```python
from build123d import *

# Parameters (mm, degrees)
SKETCH1_R           = 3.175
BOSS_EXTRUDE1_DEPTH = 27.686
SKETCH2_R           = 3.175
SKETCH2_R_2         = 2.38125
CUT_EXTRUDE1_DEPTH  = 4.318
SKETCH3_R           = 2.38125
SKETCH3_R_2         = 2.2225
CUT_EXTRUDE2_DEPTH  = 0.4572
SKETCH4_R           = 1.5875
CUT_EXTRUDE3_DEPTH  = 56.553754455


with BuildPart() as part:
    # Sketch1 → Boss-Extrude1 (new, symmetric)
    with BuildSketch(Plane.XY):
        Circle(SKETCH1_R)
    extrude(amount=BOSS_EXTRUDE1_DEPTH, both=True)

    # Sketch2 → Cut-Extrude1 (cut)
    with BuildSketch(Plane.XY.offset(27.686)):
        Circle(SKETCH2_R)
        Circle(SKETCH2_R_2, mode=Mode.SUBTRACT)
    cut_extrude1 = extrude(amount=-CUT_EXTRUDE1_DEPTH, mode=Mode.SUBTRACT)

    # Sketch3 → Cut-Extrude2 (cut)
    with BuildSketch(Plane.XY.offset(26.797)):
        Circle(SKETCH3_R)
        Circle(SKETCH3_R_2, mode=Mode.SUBTRACT)
    cut_extrude2 = extrude(amount=-CUT_EXTRUDE2_DEPTH, mode=Mode.SUBTRACT)

    # Sketch4 → Cut-Extrude3 (cut, through all)
    with BuildSketch(Plane.XY.offset(27.686)):
        Circle(SKETCH4_R)
    extrude(amount=-CUT_EXTRUDE3_DEPTH, mode=Mode.SUBTRACT)

    # Mirror1: Cut-Extrude1, Cut-Extrude2 across plane
    add(cut_extrude1.mirror(Plane.XY), mode=Mode.SUBTRACT)
    add(cut_extrude2.mirror(Plane.XY), mode=Mode.SUBTRACT)


solid = part.part
```
Geometry check sheet. Reference: the model listing, model coordinates, mm. A direction names the side the tool comes from. Give positions to 0.01 mm unless a question says otherwise; leave off trailing zeros.
1. Thickness scan on L1, parallel to Z at x = -2.25, y = 0.25; L2, parallel to Y at x = 0, z = 6 (1 decimal); L3, parallel to Y at x = 2.75, z = 7. Record the ranges inside material, lowest first.
2. Gauge pin test, flat ends, axial feed: pin 1 Ø2.5 at (x, y) = (0, 0) entering from +Z; pin 2 Ø1.5 at (x, z) = (-2.5, -20.5) entering from -Y; pin 3 Ø1 at (y, z) = (1.5, 2.5) entering from -X. Record the tip position at first contact, or that the pin passes through.
3. Access from +Z, -Z, +X, -X, +Y, -Y to the whole of each face (thin tool, end or side, straight path). Record for faces 1 (the face through (-1.89, -1.45, 27.25)), 2 (the face through (-0.48, -2.17, 26.57)), 3 (the face through (-1.89, -1.45, -24.87)).
4. Release check for a two-part mould opening along Y. For faces 4 (the face through (-0.34, -1.55, 0.39)), 5 (the face through (-1.89, -1.45, -27.25)), 6 (the face through (2, 0, 27.686)) record: pulls with the +Y half, pulls with the -Y half, needs draft (parallel to the pull), parting line crosses it, or undercut.
Values follow:
1. L1: z = -27.69 to -26.8, -26.34 to 26.34, 26.8 to 27.69
1. L2: y = -3.2 to -1.6, 1.6 to 3.2
1. L3: y = -1.59 to 1.59
2. pin 1: passes through
2. pin 2: stops at y = -2.65
2. pin 3: stops at x = -3.01
3. face 1: +Z
3. face 2: none
3. face 3: -Z
4. face 4: undercut
4. face 5: parting line crosses it
4. face 6: needs draft
